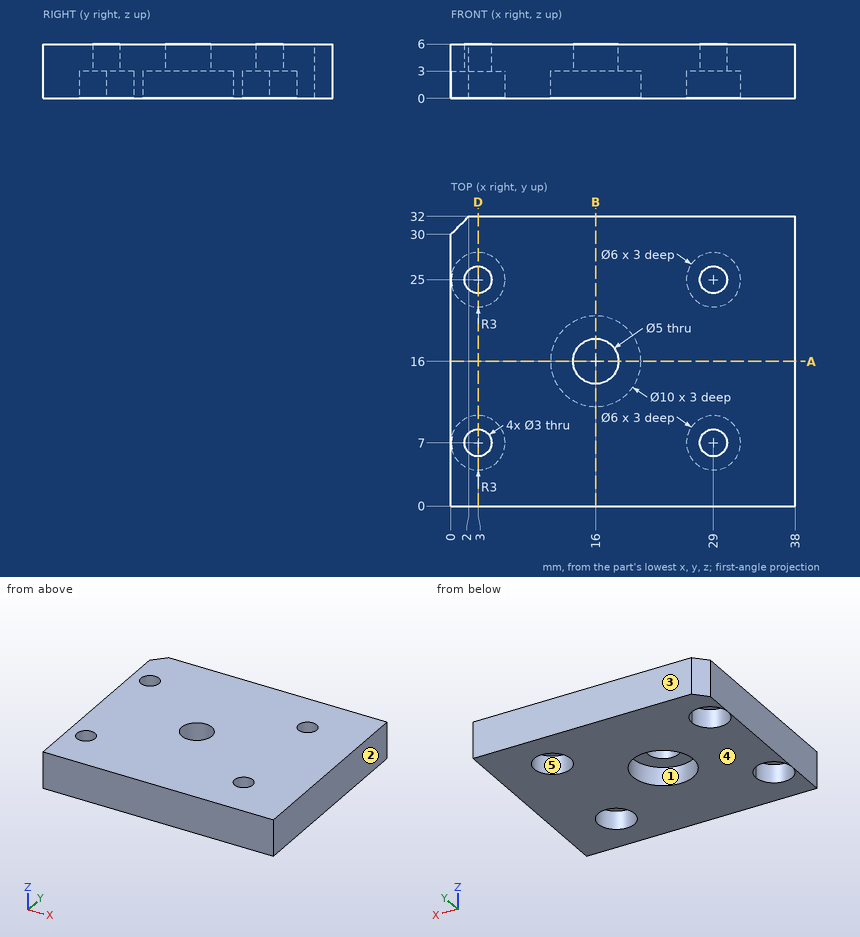
Could you check a few things on this drawing? It's one solid part, dimensions in mm from its lowest x, y, z. A direction names the side the tool comes from. Coordinates: 2 decimals unless noted, no trailing zeros. Order: outer loops, then holes, each group sorted by start corner. A loop starts at its lowest first (then second) coordinate and runs counter-clockwise, first axis right, second up.
1) Which directions (+Z, -Z, +X, -X, +Y, -Y) give clear straight access to the entire face, cutting with the end or side of a thin tool? Please do the marked faces 4 and 5.
2) Imagine slicing it at D-D on x = 3. List the corners of the cut face in (y, z) for me, and give its area (3 significant figures).
3) We'd pull the mould along X, two halves only. Please class the marked faces 1, 2 and 3: +X half, -X half, draft (parallel to the pull), parting line (faces both ways), or undercut.
4) Will these pins go through, and if not, where does the flat tip stop? pin 1 (1.8 mm diameter, centred on x = 3, y = 7, fed in from +Z); pin 2 (3.5 mm diameter, centred on x = 29, y = 25, fed in from -Z).
5) Imagine slicing it at A-A on y = 16. List the corners of the cut face in (x, z) for me, and give its area (3 significant figures).
6) I need wall thicknesses on line 1 (X direction, y = 7, z = 5); line 2 (Y direction, x = 29, z = 2.4); line 3 (Y direction, x = 30, z = 2.15). Which ranges of each line are inside material? Lowest first, please.
7) Imagine slicing it at B-B on x = 16. List the corners of the cut face in (y, z) for me.
Response values:
1. face 4: -Z, +X, -X, +Y, -Y
1. face 5: -Z
2. outline: (0, 0) - (4, 0) - (4, 3) - (5.5, 3) - (5.5, 6) - (0, 6) - close; (8.5, 3) - (10, 3) - (10, 0) - (22, 0) - (22, 3) - (23.5, 3) - (23.5, 6) - (8.5, 6) - close; (26.5, 3) - (28, 3) - (28, 0) - (32, 0) - (32, 6) - (26.5, 6) - close
2. area: 138 mm2
3. face 1: undercut
3. face 2: +X half
3. face 3: draft
4. pin 1: passes through
4. pin 2: stops at z = 3
5. outline: (0, 0) - (11, 0) - (11, 3) - (13.5, 3) - (13.5, 6) - (0, 6) - close; (18.5, 3) - (21, 3) - (21, 0) - (38, 0) - (38, 6) - (18.5, 6) - close
5. area: 183 mm2
6. line 1: x = 0 to 1.5, 4.5 to 27.5, 30.5 to 38
6. line 2: y = 0 to 4, 10 to 22, 28 to 32
6. line 3: y = 0 to 4.17, 9.83 to 22.17, 27.83 to 32
7. outline: (0, 0) - (11, 0) - (11, 3) - (13.5, 3) - (13.5, 6) - (0, 6) - close; (18.5, 3) - (21, 3) - (21, 0) - (32, 0) - (32, 6) - (18.5, 6) - close
